from build123d import *

# Parameters (mm, degrees)
F1_W     = 30
F1_H     = 160
F2_DEPTH = 160
F3_R     = 2
F4_W     = 30
F4_H     = 158
F4_H_2   = 2
F5_DEPTH = 30.001
F4_R     = 5.5
F6_DEPTH = 15


with BuildPart() as f2:
    # F1 (on face) → F2 (new body, symmetric)
    with BuildSketch(Plane.XY):
        Rectangle(F1_W, F1_H)
    extrude(amount=F2_DEPTH, both=True)

    # F3
    f3_edges = [f2.edges().sort_by_distance(p)[0] for p in [
        (15, 0, -160),
        (15, 80, 0),
        (15, 0, 160),
        (15, -80, 0),
        (-15, 80, 0),
        (-15, 0, -160),
        (-15, -80, 0),
        (-15, 0, 160),
        (0, 80, -160),
        (0, -80, -160),
        (0, 80, 160),
        (0, -80, 160),
    ]]
    fillet(f3_edges, radius=F3_R)

    # F4 (on face) → F5 (cut, through all)
    with BuildSketch(Plane.YZ.offset(15)):
        with Locations((-35, -79)):
            Rectangle(F4_W, F4_H)
        with Locations((-35, -159)):
            Rectangle(F4_W, F4_H_2)
    extrude(amount=-F5_DEPTH, mode=Mode.SUBTRACT)

    # F4 (on face) → F6 (cut)
    with BuildSketch(Plane.YZ.offset(15)):
        with Locations((60, -140)):
            Circle(F4_R)
        with Locations((0, -140)):
            Circle(F4_R)
        with Locations((0, -80)):
            Circle(F4_R)
        with Locations((60, -80)):
            Circle(F4_R)
    extrude(amount=-F6_DEPTH, mode=Mode.SUBTRACT)


solid = f2.part
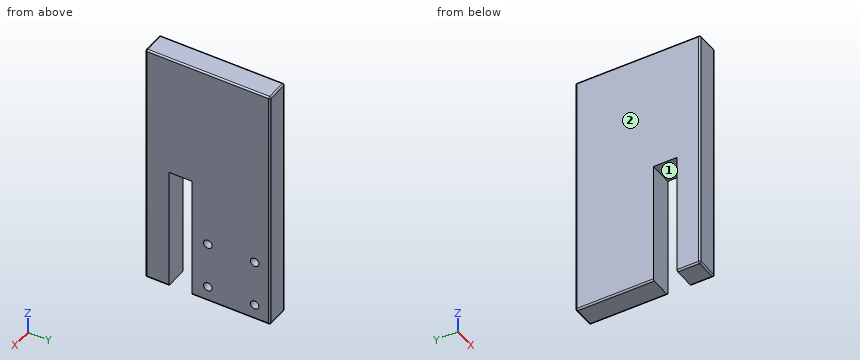
The model under review builds one solid part; all positions refer to its coordinate system, in mm. Face numbers are marked on the shaded views. A direction names the side the tool comes from. Give positions to 0.01 mm unless a question says otherwise; leave off trailing zeros. Order: outer loops, then holes, each group sorted by start corner. A loop starts at its lowest first (then second) coordinate and runs counter-clockwise, first axis right, second up. Notation, with made-up numbers: M -19,47 L 4,47 A21 ccw 4,51 Z; hole C 64,0.25 d10. An arc over 180 degrees is marked long. Use one line per item in the form item = value. Start each with the question number.
Item 1: We need section A-A on z = -80. Give the boundary of the cut face in (x, y).
Item 2: For the marked faces 1 and 2, list the 3-axis set-ups (+Z, -Z, +X, -X, +Y, -Y) from which the entire face can be reached by the end or side of a thin tool; tool diameter is ignored.
Item 3: We need section C-C on y = 0. Give the boundary of the cut face in (x, z), plus the area to 3 significant figures.
Item 4: To check wall thickness, follow line 1 along Z through (x, y) = (7, 60); line 2 along Y through (x, z) = (-5, -75.5); line 3 along X through (y, z) = (60, -135.5). State the ranges of each line that lie inside material, in increasing order. Write a range as from..to.
Item 5: We need section B-B on x = 5.5. Give the boundary of the cut face in (y, z), plus the area to 3 significant figures.
Item 6: Insertion check: pin 1 Ø5.5 at (y, z) = (61, -141) entering from +X; pin 2 Ø15 at (x, y) = (-2.5, -32) entering from -Z. Each pin has a flat end and moves straight along its axis. Give the tip position at first contact, or say it passes through.
Completed:
q1.outline = M -15,-78 A2 ccw -13,-80 L 13,-80 A2 ccw 15,-78 L 15,-50 L -15,-50 Z; M -15,-20 L 15,-20 L 15,-5.5 L 0,-5.5 L 0,5.5 L 15,5.5 L 15,54.5 L 0,54.5 L 0,65.5 L 15,65.5 L 15,78 A2 ccw 13,80 L -13,80 A2 ccw -15,78 Z
q2.face_1 = -Z, +X, -X
q2.face_2 = +Z, -Z, -X, +Y, -Y
q3.outline = M -15,-158 A2 ccw -13,-160 L 13,-160 A2 ccw 15,-158 L 15,-145.5 L 0,-145.5 L 0,-134.5 L 15,-134.5 L 15,-85.5 L 0,-85.5 L 0,-74.5 L 15,-74.5 L 15,158 A2 ccw 13,160 L -13,160 A2 ccw -15,158 Z
q3.area = 9,270 mm²
q4.line_1 = -160..-145.5, -134.5..-85.5, -74.5..160
q4.line_2 = -80..-50, -20..80
q4.line_3 = -15..0
q5.outline = M -80,-158 A2 ccw -78,-160 L -50,-160 L -50,0 L -20,0 L -20,-160 L 78,-160 A2 ccw 80,-158 L 80,158 A2 ccw 78,160 L -78,160 A2 ccw -80,158 Z; hole C 0,-140 d11; hole C 0,-80 d11; hole C 60,-140 d11; hole C 60,-80 d11
q5.area = 46,000 mm²
q6.pin_1 = 0
q6.pin_2 = 0
